Check sheet for the modelled part. Datum: model origin and axes. Units: mm. Round coordinates to 2 decimals unless told otherwise and drop trailing zeros. Write each loop counter-clockwise with the first axis right and the second up, starting at its lowest first coordinate (ties: lowest second). Pieces come first, ordered by that corner, then holes. Notation, with made-up numbers: (89.25, -1.75) -> (111.25, -1.75) arc R17 ccw to (111.25, 15.25) -> close; hole circle Ø6 at (-1, 69). An arc over 180 degrees is marked (long way). One line per item, written item: value.
Autodesk Inventor part; units mm, degrees
ref_plane "YZ Plane" through (0, 0, 0) normal (1, 0, 0) x (0, 1, 0)
ref_plane "XZ Plane" through (0, 0, 0) normal (0, 1, 0) x (-1, 0, 0)
ref_plane "XY Plane" through (0, 0, 0) normal (0, 0, 1) x (1, 0, 0)
sketch "スケッチ1" plane through (0, 0, 0) normal (0, 0, 1) x (1, 0, 0)
  line L0 (1.5437, -2.775) -> (-1.6314, -2.7243)
  line L1 (-1.6314, -2.7243) -> (-3.175, 0.0506)
  line L2 (-3.175, 0.0506) -> (-1.5437, 2.775)
  line L3 (-1.5437, 2.775) -> (1.6314, 2.7243)
  line L4 (1.6314, 2.7243) -> (3.175, -0.0506)
  line L5 (3.175, -0.0506) -> (1.5437, -2.775)
  point P0 (0, 0)
  point P1 (0, 0)
  dimension "d0" = 5.5
extrude "押し出し1" add sketch "スケッチ1" along normal blind 2.4
sketch "スケッチ2" plane through (0, 0, 2.4) normal (0, 0, 1) x (1, 0, 0)
  circle A0 centre (0, 0) radius 1.5
  dimension "d3" = 3
extrude "押し出し2" cut sketch "スケッチ2" against normal blind 2.4
thread "ねじ1"
chamfer "面取り1" distance 0.5 angle 45 12 edges at (2.3593, -1.4128, 2.4) (2.4032, 1.3369, 2.4) (0.0438, 2.7497, 2.4) (-2.3593, 1.4128, 2.4) (-2.4032, -1.3369, 2.4) (-0.0438, -2.7497, 2.4) (-0.0438, -2.7497, 0) (2.3593, -1.4128, 0) (2.4032, 1.3369, 0) (0.0438, 2.7497, 0) (-2.3593, 1.4128, 0) (-2.4032, -1.3369, 0)
properties part number "Nut" material "真鍮"
Item 1: Sectioned sample at A-A (y = 0.8). Enter the section's corners in (x, z).
Result set:
outline: (-2.73, 0.5) -> (-2.14, 0) -> (-1.27, 0) -> (-1.27, 2.4) -> (-2.14, 2.4) -> (-2.73, 1.9) -> close; (1.27, 0) -> (2.13, 0) -> (2.7, 0.5) -> (2.7, 1.9) -> (2.13, 2.4) -> (1.27, 2.4) -> close
Item 2: Depth check by flat-ended pin: pin 1 (3 mm diameter, centred on x = 1, y = 0, fed in from +Z); pin 2 (1 mm diameter, centred on x = 0, z = 1, fed in from +Y); pin 3 (1 mm diameter, centred on x = 1.5, z = 1.5, fed in from +Y). Enter the tip coordinate at first touch or a pass-through.
Result set:
pin 1: z = 2.4
pin 2: y = 2.76
pin 3: y = 2.73
Item 3: Release check for a two-part mould opening along Y. For faces 1 (the cylindrical face through (-1.5, 0.07, 1.22)), 2 (the flat face through (0, 2, 0)), 3 (the flat face through (2.177, 1.236, 2.147)), 4 (the flat face through (2.13, -1.302, 2.153)) record: pulls with the +Y half, pulls with the -Y half, needs draft (parallel to the pull), parting line crosses it, or undercut.
Result set:
face 1: undercut
face 2: needs draft
face 3: pulls with the +Y half
face 4: pulls with the -Y half
Item 4: Sectioned sample at C-C (x = 0). Enter the section's corners in (y, z), then the cut area to 3 significant figures.
Result set:
outline: (-2.75, 0.5) -> (-2.25, 0) -> (-1.5, 0) -> (-1.5, 2.4) -> (-2.25, 2.4) -> (-2.75, 1.9) -> close; (1.5, 0) -> (2.25, 0) -> (2.75, 0.5) -> (2.75, 1.9) -> (2.25, 2.4) -> (1.5, 2.4) -> close
area: 5.50 mm^2
Item 5: Material ranges on line 1 along X through (y, z) = (0.2, 1.95); line 2 along Y through (x, z) = (0, 0.6); line 3 along X through (y, z) = (-0.4, 1.45), recorded low to high.
Result set:
line 1: -3.03 to -1.49, 1.49 to 2.98
line 2: -2.75 to -1.5, 1.5 to 2.75
line 3: -2.92 to -1.45, 1.45 to 2.97
Item 6: Sectioned sample at D-D (z = 2.2). Enter the section's corners in (x, y), then the cut area to 3 significant figures.
Result set:
outline: (-2.83, 0.05) -> (-1.45, -2.43) -> (1.38, -2.47) -> (2.83, -0.05) -> (1.45, 2.43) -> (-1.38, 2.47) -> close; hole circle Ø3 at (0, 0)
area: 13.7 mm^2
Item 7: Sectioned sample at B-B (z = 0.75). Enter the section's corners in (x, y) (3 decimals), then the cut area to 3 significant figures.
Result set:
outline: (-3.175, 0.051) -> (-1.631, -2.724) -> (1.544, -2.775) -> (3.175, -0.051) -> (1.631, 2.724) -> (-1.544, 2.775) -> close; hole circle Ø3 at (0, 0)
area: 19.1 mm^2
